```python
from build123d import *

# Parameters (mm, degrees)
SKETCH4_R           = 42.545
BOSS_EXTRUDE2_DEPTH = 0.254
SKETCH5_R           = 29.845
CUT_EXTRUDE5_DEPTH  = 1.254
CUT_EXTRUDE6_DEPTH  = 1.254
CUT_EXTRUDE11_DEPTH = 1.254


with BuildPart() as part:
    # Sketch4 → Boss-Extrude2 (new body)
    with BuildSketch(Plane.XY):
        Circle(SKETCH4_R)
    extrude(amount=BOSS_EXTRUDE2_DEPTH)

    # Sketch5 → Cut-Extrude5 (cut, through all)
    with BuildSketch(Plane.XY.offset(0.254)):
        Circle(SKETCH5_R)
    extrude(amount=-CUT_EXTRUDE5_DEPTH, mode=Mode.SUBTRACT)

    # Sketch6 → Cut-Extrude6 (cut, through all)
    with BuildSketch(Plane.XY.offset(0.254)):
        with BuildLine():
            ThreePointArc((28.916424965, 28.916424455), (22.27103521, 28.916424739), (22.271035377, 22.271034984))
            ThreePointArc((22.271035377, 22.271034984), (29.098509704, 12.052997511), (31.496, 5.5e-07))
            ThreePointArc((31.496, 5.5e-07), (36.195000082, -4.699), (40.894, 7.14e-07))
            ThreePointArc((40.894, 7.14e-07), (37.781129535, 15.649456446), (28.916424965, 28.916424455))
        make_face()
        with BuildLine():
            ThreePointArc((28.916424455, -28.916424965), (28.916424739, -22.27103521), (22.271034984, -22.271035377))
            ThreePointArc((22.271034984, -22.271035377), (12.052997511, -29.098509704), (5.5e-07, -31.496))
            ThreePointArc((5.5e-07, -31.496), (-4.699, -36.195000082), (7.14e-07, -40.894))
            ThreePointArc((7.14e-07, -40.894), (15.649456446, -37.781129535), (28.916424455, -28.916424965))
        make_face()
        with BuildLine():
            ThreePointArc((-28.916424965, -28.916424455), (-22.27103521, -28.916424739), (-22.271035377, -22.271034984))
            ThreePointArc((-22.271035377, -22.271034984), (-29.098509704, -12.052997511), (-31.496, -5.5e-07))
            ThreePointArc((-31.496, -5.5e-07), (-36.195000082, 4.699), (-40.894, -7.14e-07))
            ThreePointArc((-40.894, -7.14e-07), (-37.781129535, -15.649456446), (-28.916424965, -28.916424455))
        make_face()
        with BuildLine():
            ThreePointArc((-28.916424455, 28.916424965), (-28.916424739, 22.27103521), (-22.271034984, 22.271035377))
            ThreePointArc((-22.271034984, 22.271035377), (-12.052997511, 29.098509704), (-5.5e-07, 31.496))
            ThreePointArc((-5.5e-07, 31.496), (4.699, 36.195000082), (-7.14e-07, 40.894))
            ThreePointArc((-7.14e-07, 40.894), (-15.649456446, 37.781129535), (-28.916424455, 28.916424965))
        make_face()
    extrude(amount=-CUT_EXTRUDE6_DEPTH, mode=Mode.SUBTRACT)

    # Sketch8 → Cut-Extrude11 (cut, through all)
    with BuildSketch(Plane.XY.offset(0.254)):
        Polygon((40.379126173, 15.350943603), (39.407110255, 17.697597616), (38.233783248, 17.211589657), (39.205799167, 14.864935644), align=None)
        Polygon((-15.350943603, 40.379126173), (-17.697597616, 39.407110255), (-17.211589657, 38.233783248), (-14.864935644, 39.205799167), align=None)
        Polygon((-39.407110255, 17.697597616), (-40.379126173, 15.350943603), (-39.205799167, 14.864935644), (-38.233783248, 17.211589657), align=None)
        Polygon((-40.379126173, -15.350943603), (-39.407110255, -17.697597616), (-38.233783248, -17.211589657), (-39.205799167, -14.864935644), align=None)
        Polygon((-17.697597616, -39.407110255), (-15.350943603, -40.379126173), (-14.864935644, -39.205799167), (-17.211589657, -38.233783248), align=None)
        Polygon((15.350943603, -40.379126173), (17.697597616, -39.407110255), (17.211589657, -38.233783248), (14.864935644, -39.205799167), align=None)
        Polygon((39.407110255, -17.697597616), (40.379126173, -15.350943603), (39.205799167, -14.864935644), (38.233783248, -17.211589657), align=None)
        Polygon((17.697597616, 39.407110255), (15.350943603, 40.379126173), (14.864935644, 39.205799167), (17.211589657, 38.233783248), align=None)
    extrude(amount=-CUT_EXTRUDE11_DEPTH, mode=Mode.SUBTRACT)


solid = part.part
```
Part model, mm, in its own coordinate system. Round coordinates to 2 decimals unless told otherwise and drop trailing zeros. Loops run counter-clockwise (first coordinate to the right, second up) from the corner with the lowest first, then second, coordinate; pieces in that order, holes last.
Item 1: Cut at B-B, the plane x = -36. Give the cut face in (y, z).
Item 2: Cut at C-C, the plane x = -9.5. Give the cut face in (y, z).
Item 3: Drill centre lines: line 1 (X direction, y = -3, z = 0.2); line 2 (X direction, y = 27.5, z = 0.15); line 3 (X direction, y = -9, z = 0.1). Where is each one in solid material? Low to high.
Item 4: Cut at A-A, the plane y = 11.5. Give the cut face in (x, z).
Item 5: Drop a flat-ended pin along its axis: P1, Ø1, axis at x = 26, y = 20, coming from the -Z side (1 decimal). Give the stop position or say it passes through.
A:
1. outline: (-22.67, 0) - (-19.4, 0) - (-19.4, 0.25) - (-22.67, 0.25) - close; (4.69, 0) - (22.67, 0) - (22.67, 0.25) - (4.69, 0.25) - close
2. outline: (-41.47, 0) - (-28.29, 0) - (-28.29, 0.25) - (-41.47, 0.25) - close; (28.29, 0) - (30.03, 0) - (30.03, 0.25) - (28.29, 0.25) - close; (39.78, 0) - (41.47, 0) - (41.47, 0.25) - (39.78, 0.25) - close
3. line 1: x = -42.44 to -40.78, -31.35 to -29.69, 29.69 to 32.58, 39.81 to 42.44
3. line 2: x = -32.46 to -29.89, -15.35 to -11.6, 11.6 to 21.3, 30.27 to 32.46
3. line 3: x = -41.58 to -39.89, -30.18 to -28.46, 28.46 to 41.58
4. outline: (-40.96, 0) - (-27.54, 0) - (-27.54, 0.25) - (-40.96, 0.25) - close; (27.54, 0) - (29.32, 0) - (29.32, 0.25) - (27.54, 0.25) - close; (39.24, 0) - (40.96, 0) - (40.96, 0.25) - (39.24, 0.25) - close
5. P1: passes through
